from build123d import *

# Parameters (mm, degrees)
SKETCH_W     = 9
SKETCH_H     = 11
PAD_DEPTH    = 3.5
PAD001_DEPTH = 10
SKETCH003_W  = 3
SKETCH003_H  = 3.5
PAD002_DEPTH = 1
SKETCH004_R  = 3
POCKET_DEPTH = 10
FILLET_R     = 0.1
FILLET002_R  = 0.1
FILLET003_R  = 0.1
FILLET004_R  = 0.1
FILLET006_R  = 0.1


with BuildPart() as part:
    # Sketch → Pad (new body)
    with BuildSketch(Plane.XZ):
        with Locations((0, -1)):
            Rectangle(SKETCH_W, SKETCH_H)
    extrude(amount=-PAD_DEPTH)

    # Sketch001 (on Face6 of Pad) → Pad001 (join)
    with BuildSketch(Plane(origin=(0, 3.5, 0), x_dir=(1, 0, 0), z_dir=(0, 1, 0))):
        with BuildLine():
            ThreePointArc((-4.3, 0), (0, -4.3), (4.3, 0))
            Line((4.3, 0), (4.5, 0))
            Line((4.5, 6.5), (4.5, 0))
            Line((-4.5, 6.5), (4.5, 6.5))
            Line((-4.5, 0), (-4.5, 6.5))
            Line((-4.5, 0), (-4.3, 0))
        make_face()
    extrude(amount=PAD001_DEPTH)

    # Sketch003 → Pad002 (join)
    with BuildSketch(Plane(origin=(0, 13.5, 0), x_dir=(1, 0, 0), z_dir=(0, 1, 0))):
        with Locations((-3, 4.75)):
            Rectangle(SKETCH003_W, SKETCH003_H)
        with Locations((3, 4.75)):
            Rectangle(SKETCH003_W, SKETCH003_H)
    extrude(amount=PAD002_DEPTH)

    # Sketch004 (on Face4 of Pad002) → Pocket (cut)
    with BuildSketch(Plane.XZ):
        Circle(SKETCH004_R)
    extrude(amount=-POCKET_DEPTH, mode=Mode.SUBTRACT)

    # Fillet
    fillet_edges = [part.edges().sort_by_distance(p)[0] for p in [
        (0, 0, 4.5),
        (4.5, 0, -1),
        (0, 0, -6.5),
        (-4.5, 0, -1),
        (0, 3.5, 4.5),
        (4.5, 3.5, 2.25),
        (-4.5, 3.5, 2.25),
    ]]
    fillet(fillet_edges, radius=FILLET_R)

    # Fillet002
    fillet002_edges = [part.edges().sort_by_distance(p)[0] for p in [
        (0, 13.5, 4.3),
    ]]
    fillet(fillet002_edges, radius=FILLET002_R)

    # Fillet003
    fillet003_edges = [part.edges().sort_by_distance(p)[0] for p in [
        (3, 14.5, -3),
        (4.5, 14.5, -4.75),
        (3, 14.5, -6.5),
        (1.5, 14.5, -4.75),
        (-1.5, 14.5, -4.75),
        (-3, 14.5, -3),
        (-4.5, 14.5, -4.75),
        (-3, 14.5, -6.5),
    ]]
    fillet(fillet003_edges, radius=FILLET003_R)

    # Fillet004
    fillet004_edges = [part.edges().sort_by_distance(p)[0] for p in [
        (-4.5, 8.5, 0),
        (4.5, 8.5, 0),
    ]]
    fillet(fillet004_edges, radius=FILLET004_R)

    # Fillet006
    fillet006_edges = [part.edges().sort_by_distance(p)[0] for p in [
        (-3, 0, 0),
    ]]
    fillet(fillet006_edges, radius=FILLET006_R)


solid = part.part
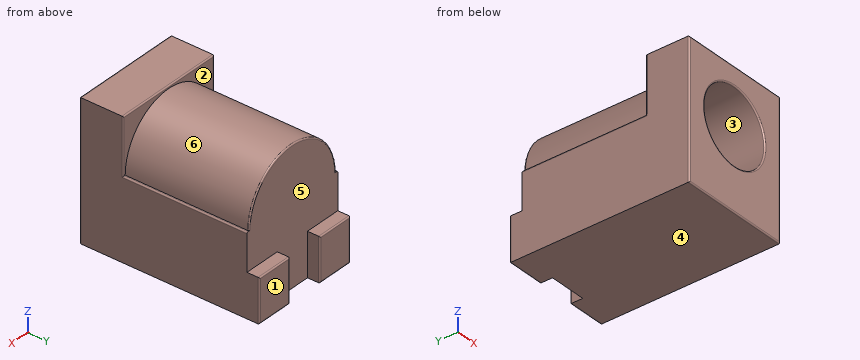
Verification items for the finished model (mm, model axes). Face numbers are marked on the shaded views. A direction names the side the tool comes from. Coordinates: 2 decimals unless noted, no trailing zeros. Loops run counter-clockwise (first coordinate to the right, second up) from the corner with the lowest first, then second, coordinate; pieces in that order, holes last. Notation, with made-up numbers: M 88,7.5 L 106,7.5 A19 ccw 106,39.5 Z; hole C 9.5,6 d6. An arc over 180 degrees is marked long. One line per item, written item: value.
1. Gauge pin test, flat ends, axial feed: P1, Ø3.5, axis at x = -1, z = 3, coming from the +Y side; P2, Ø1.8, axis at x = -1, z = 1, coming from the -Y side; P3, Ø0.5, axis at x = -3, y = 14, coming from the +Z side. Record the tip position at first contact, or that the pin passes through.
Answers follow:
P1: y = 13.5
P2: y = 10
P3: z = -3
2. Section check C-C on x = 0. Record the cut outline in (y, z), plus the area to 3 significant figures.
Answers follow:
outline: M 0,-6.4 A0.1 ccw 0.1,-6.5 L 13.5,-6.5 L 13.5,4.2 A0.1 ccw 13.4,4.3 L 3.5,4.3 L 3.5,4.4 A0.1 ccw 3.4,4.5 L 0.1,4.5 A0.1 ccw 0,4.4 L 0,3.1 A0.1 ccw 0.1,3 L 10,3 L 10,-3 L 0.1,-3 A0.1 ccw 0,-3.1 Z
area: 86.5 mm^2
3. Set-up check for the marked faces 1 and 2: record each of +Z, -Z, +X, -X, +Y, -Y from which the full face is reachable in a straight line by a thin tool's end or side.
Answers follow:
face 1: +Z, -Z, +X, -X, +Y
face 2: +Z, +Y
4. Section check B-B on z = -3.5. Record the cut outline in (x, y), plus the area to 3 significant figures.
Answers follow:
outline: M -4.5,0.1 A0.1 ccw -4.4,0 L 4.4,0 A0.1 ccw 4.5,0.1 L 4.5,14.4 A0.1 ccw 4.4,14.5 L 1.6,14.5 A0.1 ccw 1.5,14.4 L 1.5,13.5 L -1.5,13.5 L -1.5,14.4 A0.1 ccw -1.6,14.5 L -4.4,14.5 A0.1 ccw -4.5,14.4 Z
area: 127 mm^2
5. Section check A-A on y = 4.5. Record the cut outline in (x, z).
Answers follow:
outline: M -4.5,-6.5 L 4.5,-6.5 L 4.5,-0.1 A0.1 ccw 4.4,0 L 4.3,0 A4.3 ccw -4.3,0 L -4.4,0 A0.1 ccw -4.5,-0.1 Z; hole C 0,0 d6
6. Material ranges on line 1 along Z through (x, y) = (0, 7); line 2 along Z through (x, y) = (0, 11.25); line 3 along Y through (x, z) = (1.25, -1), recorded low to high. Write a range as from..to.
Answers follow:
line 1: -6.5..-3, 3..4.3
line 2: -6.5..4.3
line 3: 10..13.5
7. Mould release check, pull along X, two halves, no side actions. Record for the marked faces 3, 4, 5 and 6: pulls with the +X half, pulls with the -X half, needs draft (parallel to the pull), parting line crosses it, or undercut.
Answers follow:
face 3: undercut
face 4: needs draft
face 5: undercut
face 6: parting line crosses it
8. Section check D-D on y = 1.5. Record the cut outline in (x, z), plus the area to 3 significant figures.
Answers follow:
outline: M -4.5,-6.5 L 4.5,-6.5 L 4.5,4.5 L -4.5,4.5 Z; hole C 0,0 d6
area: 70.7 mm^2
